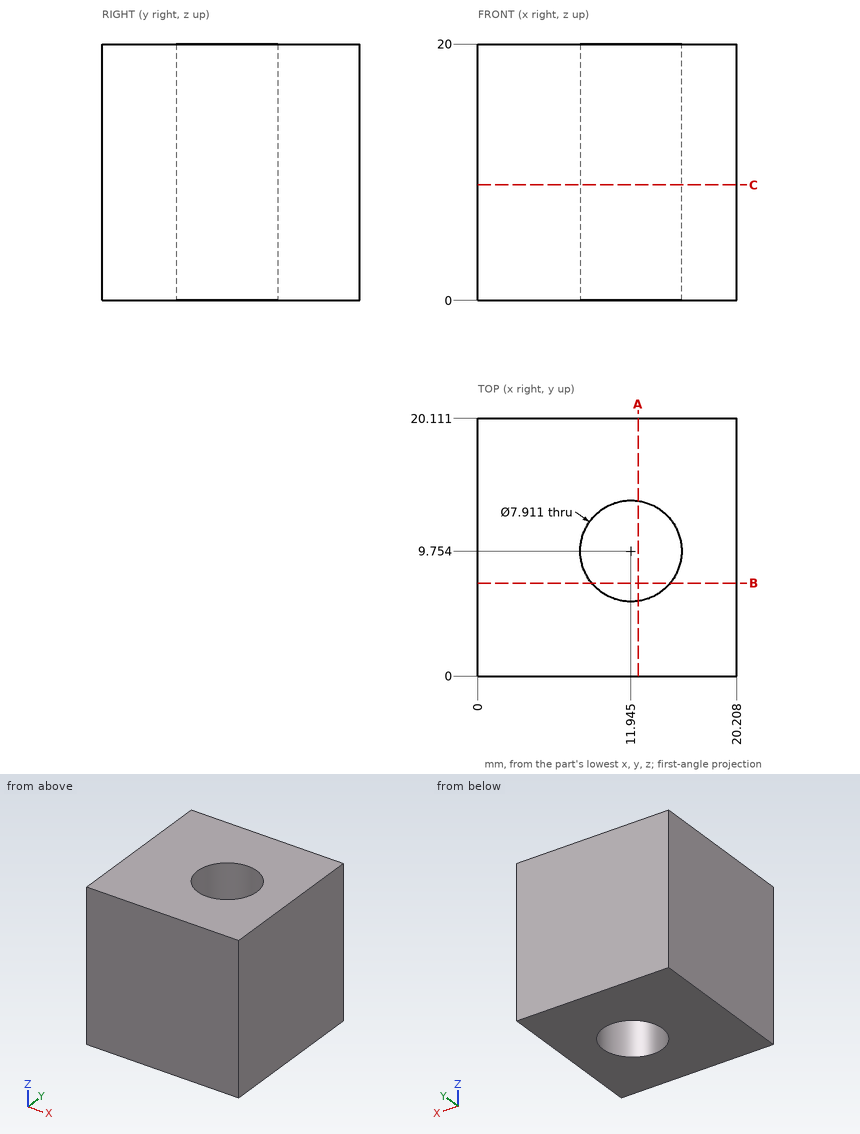
Answer from the drawing. Dimensions are ordinates in mm from the lowest x, y and z of the part. Coordinates: 2 decimals unless noted, no trailing zeros. Loops run counter-clockwise (first coordinate to the right, second up) from the corner with the lowest first, then second, coordinate; pieces in that order, holes last.
1) Section A-A (x = 12.5) is taken. Give the vertices of the cut face in (y, z).
Results:
outline: (0, 0) - (5.84, 0) - (5.84, 20) - (0, 20) - close; (13.67, 0) - (20.11, 0) - (20.11, 20) - (13.67, 20) - close
2) Consider probe 1 along X at (y, z) = (11.75, 19); probe 2 along Y at (x, z) = (12.5, 12); probe 3 along Y at (x, z) = (9, 6.5) (1 decimal). Determine where each line is inside the solid, lowest interval first.
Results:
probe 1: x = 0 to 8.53, 15.36 to 20.21
probe 2: y = 0 to 5.84, 13.67 to 20.11
probe 3: y = 0 to 7.1, 12.4 to 20.1
3) Section C-C (z = 9) is taken. Give the vertices of the cut face in (x, y) (1 decimal).
Results:
outline: (0, 0) - (20.2, 0) - (20.2, 20.1) - (0, 20.1) - close; hole circle Ø7.9 at (11.9, 9.8)
4) Section B-B (y = 7.25) is taken. Give the vertices of the cut face in (x, z), plus the area to 3 significant figures.
Results:
outline: (0, 0) - (8.88, 0) - (8.88, 20) - (0, 20) - close; (15.01, 0) - (20.21, 0) - (20.21, 20) - (15.01, 20) - close
area: 282 mm2
